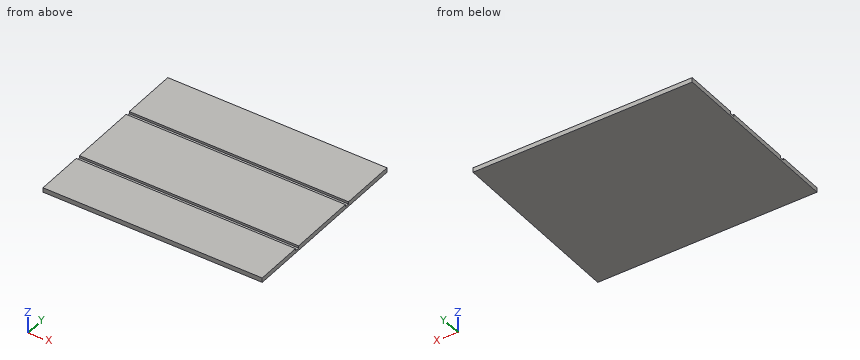
from build123d import *

# Parameters (mm, degrees)
F0_W     = 762
F0_H     = 19.05
F1_DEPTH = 914.4
F2_W     = 19.05
F2_H     = 9.525
F3_DEPTH = 914.401
F4_W     = 38.1
F4_H     = 38.1
F5_DEPTH = 711.2


with BuildPart() as f1:
    # F0 (on Right) → F1 (new body)
    with BuildSketch(Plane.YZ):
        with Locations((381, 9.525)):
            Rectangle(F0_W, F0_H)
    extrude(amount=-F1_DEPTH)

    # F2 (on face) → F3 (cut, through all)
    with BuildSketch(Plane.YZ):
        with Locations((212.725, 14.2875)):
            Rectangle(F2_W, F2_H)
        with Locations((517.525, 14.2875)):
            Rectangle(F2_W, F2_H)
    extrude(amount=-F3_DEPTH, mode=Mode.SUBTRACT)


with BuildPart() as f5:
    # F4 (on face) → F5 (new body)
    with BuildSketch(Plane(origin=(0, 0, 0), x_dir=(1, 0, 0), z_dir=(0, 0, -1))):
        with Locations((-895.35, -31.75)):
            Rectangle(F4_W, F4_H)
    extrude(amount=F5_DEPTH)


solid = f1.part
Source: CAD feature listing. Evaluate the final solid. Frame: model axes, mm. Round coordinates to 2 decimals unless told otherwise and drop trailing zeros. Loops run counter-clockwise (first coordinate to the right, second up) from the corner with the lowest first, then second, coordinate; pieces in that order, holes last. Notation, with made-up numbers: (78, 31) -> (89, 31) arc R17 cw to (89, 42) -> close; hole circle Ø9 at (44, -36.75). An arc over 180 degrees is marked (long way). Answer as a JSON object with one key per item and string values. Group by question number.
Q1. Section query A-A (z = 13.5). Output: boundary loops of the cut face in (x, y), plus the area to 3 significant figures.
Q2. Contact query for flat-ended pins moving along their axis: P1, Ø1.5, axis at x = -519.5, z = 16, coming from the -Y side; P2, Ø5.5, axis at x = -443.5, y = 215, coming from the +Z side (3 decimals). Output: stop coordinate, or through.
Q3. Section query B-B (x = -553). Output: boundary loops of the cut face in (y, z) (3 decimals), plus the area to 3 significant figures.
Q4. Ray query, line 1 (Y direction, x = -542, z = 18.25); line 2 (Z direction, x = -69, y = 512.5) (3 decimals). Return the intervals inside material, ascending. Write a range as from..to.
Completed:
{
 "1": {"outline": "(-914.4, 0) -> (0, 0) -> (0, 203.2) -> (-914.4, 203.2) -> close; (-914.4, 222.25) -> (0, 222.25) -> (0, 508) -> (-914.4, 508) -> close; (-914.4, 527.05) -> (0, 527.05) -> (0, 762) -> (-914.4, 762) -> close", "area": "662,000 mm²"},
 "2": {"P1": "y = 0", "P2": "z = 9.525"},
 "3": {"outline": "(0, 0) -> (762, 0) -> (762, 19.05) -> (527.05, 19.05) -> (527.05, 9.525) -> (508, 9.525) -> (508, 19.05) -> (222.25, 19.05) -> (222.25, 9.525) -> (203.2, 9.525) -> (203.2, 19.05) -> (0, 19.05) -> close", "area": "14,200 mm²"},
 "4": {"line 1": "0..203.2, 222.25..508, 527.05..762", "line 2": "0..9.525"}
}
